Here's how the part is built. I have some questions about the finished solid (model axes, mm). Face numbers are marked on the shaded views. A direction names the side the tool comes from. Coordinates: 2 decimals unless noted, no trailing zeros. Write each loop counter-clockwise with the first axis right and the second up, starting at its lowest first coordinate (ties: lowest second). Pieces come first, ordered by that corner, then holes. Notation, with made-up numbers: M -17,20.5 L 38,20.5 A15 cw 38,44.5 Z; hole C -28.5,42 d2. An arc over 180 degrees is marked long. Use one line per item in the form item = value. Start each with the question number.
1. On a 3-axis mill with a long thin cutter (end or side, diameter ignored), from which of +Z, -Z, +X, -X, +Y, -Y can I reach the whole of each face in a straight line? I mean the marked faces 1, 2 and 3. Say none if no direction works.
2. Please list where these lines run through material, in increasing order: line 1 along Z through (x, y) = (10, 2.3); line 2 along X through (y, z) = (1.6, 13.5); line 3 along Z through (x, y) = (-9, 2.7). Write a range as [from, to].
3. I want a section at A-A, the plane z = -13.5. Count the separate pieces of the cut face and the enclosed holes in it, plus the area to 3 significant figures.
4. I want a section at B-B, the plane x = -9.75. List the corners of the cut face in (y, z) for me, plus the area to 3 significant figures.
5. I want a section at D-D, the plane x = 13.5. List the corners of the cut face in (y, z) for me.
6. I'm going to push flat-ended pins straight in: pin 1 Ø3 at (x, z) = (7.5, -5.5) entering from +Y; pin 2 Ø4.5 at (x, z) = (10, -13.5) entering from -Y. Where does each tip first touch, or does it pass through?
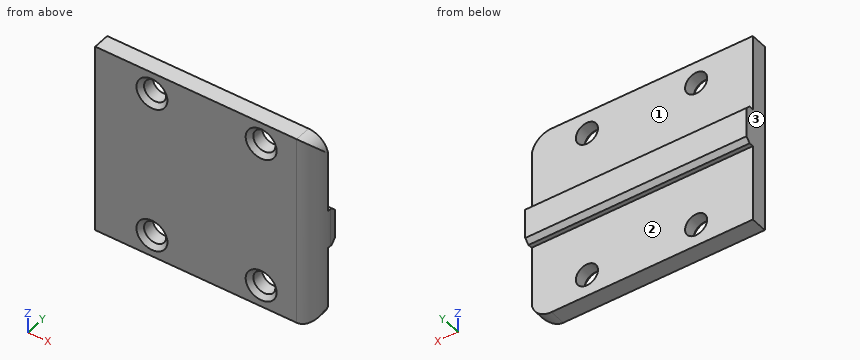
Autodesk Inventor part; units mm, degrees
ref_plane "YZ Plane" through (0, 0, 0) normal (1, 0, 0) x (0, 1, 0)
ref_plane "XZ Plane" through (0, 0, 0) normal (0, 1, 0) x (-1, 0, 0)
ref_plane "XY Plane" through (0, 0, 0) normal (0, 0, 1) x (1, 0, 0)
sketch "Sketch2" plane through (0, 0, 0) normal (0, 1, 0) x (-1, 0, 0)
  line L0 (20, 17.5) -> (-20, 17.5)
  line L1 (-20, 17.5) -> (-20, -17.5)
  line L2 (-20, -17.5) -> (20, -17.5)
  line L3 (20, -17.5) -> (20, 17.5)
  point P0 (0, 0)
  point P1 (20, 0)
  point P2 (0, -17.5)
  dimension "d0" = 40
  dimension "d1" = 35
extrude "Extrusion1" add sketch "Sketch2" along normal blind 3
sketch "Sketch3" plane through (0, 3, 0) normal (0, 1, 0) x (1, 0, 0)
  line L0 (-20, -17.5) -> (20, -17.5)
  line L1 (20, -17.5) -> (20, 17.5)
  line L2 (20, 17.5) -> (-20, 17.5)
  line L3 (-20, 17.5) -> (-20, -17.5)
  line L4 (-20, 0) -> (20, 0)
  line L5 (0, 0) -> (-9.75, 0)
  line L6 (-9.75, 0) -> (-9.75, 17.5)
  line L7 (0, 0) -> (9.75, 0)
  line L8 (9.75, 0) -> (9.75, 17.5)
  line L9 (0, 0) -> (0, 13.5)
  line L10 (0, 13.5) -> (-20, 13.5)
  line L11 (0, 13.5) -> (20, 13.5)
  circle A0 centre (10, 13.5) radius 2
  circle A1 centre (-9.75, 13.5) radius 2
  circle A2 centre (10, -13.5) radius 2
  circle A3 centre (-9.75, -13.5) radius 2
  dimension "d4" = 9.75
  dimension "d5" = 9.75
  dimension "d6" = 13.5
  dimension "d7" = 4
  dimension "d8" = 4
extrude "Extrusion2" cut sketch "Sketch3" against normal through all contours A1 L6 L10 | L10 L6 A1 | L6 L10 A1 | A0 L8 L11 | L11 L8 A0 | A0 L11 L8 | L6 A1 L10 | L11 A0 L8 | A2 | A3
sketch "Sketch4" plane through (0, 3, 0) normal (0, 1, 0) x (1, 0, 0)
  circle A0 centre (10, -13.5) radius 2
  circle A1 centre (-9.75, 13.5) radius 2
  circle A2 centre (10, 13.5) radius 2
  circle A3 centre (-9.75, -13.5) radius 2
  line L0 (-20, -17.5) -> (20, -17.5)
  line L1 (20, -17.5) -> (20, 17.5)
  line L2 (20, 17.5) -> (-20, 17.5)
  line L3 (-20, 17.5) -> (-20, -17.5)
  line L4 (20, -3.5) -> (-20, -3.5)
  line L5 (-20, -3.5) -> (-20, 3.5)
  line L6 (-20, 3.5) -> (20, 3.5)
  line L7 (20, 3.5) -> (20, -3.5)
  line L8 (20, -3.5) -> (-20, 3.5) construction
  line L9 (-20, -3.5) -> (20, 3.5) construction
  point P0 (0, 0)
  dimension "d11" = 7
extrude "Extrusion3" add sketch "Sketch4" along normal blind 1.6 contours L3 L6 L1 L4
fillet "Fillet1" radius 3.5875 3 edges at (20, 1.5, 17.5) (20, 1.5, -17.5) (20, 0, 0)
sketch "Sketch5" plane through (0, 0, 0) normal (0, -1, 0) x (1, 0, 0)
  circle A0 centre (-9.75, 13.5) radius 2
  circle A1 centre (10, -13.5) radius 2
  circle A2 centre (-9.75, -13.5) radius 2
  circle A3 centre (10, 13.5) radius 2
  line L0 (16.4125, 17.5) -> (16.4125, -17.5)
  line L1 (-20, 17.5) -> (16.4125, 17.5)
  line L2 (-20, -17.5) -> (-20, 17.5)
  line L3 (16.4125, -17.5) -> (-20, -17.5)
  circle A4 centre (-9.75, 13.5) radius 3
  circle A5 centre (10, 13.5) radius 3
  circle A6 centre (10, -13.5) radius 3
  circle A7 centre (-9.75, -13.5) radius 3
  point P0 (0, 0)
  dimension "d15" = 1
  dimension "d16" = 1
  dimension "d17" = 1
  dimension "d18" = 1
chamfer "Chamfer1" distance 0.8 angle 45 4 edges at (-11.75, 0, -13.5) (-11.75, 0, 13.5) (8, 0, 13.5) (8, 0, -13.5)
chamfer "Chamfer2" distance 0.8 angle 45 2 edges at (0, 4.6, 3.5) (0, 4.6, -3.5)
properties part number "RearCarriageSupport" material "ABS Plastic"
Answer list:
q1.face_1 = +Z, +X, -X, +Y
q1.face_2 = -Z, +X, -X, +Y
q1.face_3 = +Z, -Z, -X, +Y, -Y
q2.line_1 = [-17.5, -15.5], [-11.5, 11.5], [15.5, 17.5]
q2.line_2 = [-20, -11.75], [-7.75, 8], [12, 19.4]
q2.line_3 = [-17.5, -15.35], [-11.65, 11.65], [15.35, 17.5]
q3.separate_pieces = 3
q3.enclosed_holes = 0
q3.area = 92.0 mm²
q4.outline = M 0,-17.5 L 3,-17.5 L 3,-15.5 L 0.8,-15.5 L 0,-16.3 Z; M 0,-10.7 L 0.8,-11.5 L 3,-11.5 L 3,-3.5 L 3.8,-3.5 L 4.6,-2.7 L 4.6,2.7 L 3.8,3.5 L 3,3.5 L 3,11.5 L 0.8,11.5 L 0,10.7 Z; M 0,16.3 L 0.8,15.5 L 3,15.5 L 3,17.5 L 0,17.5 Z
q4.area = 90.3 mm²
q5.outline = M 0,-17.5 L 3,-17.5 L 3,-3.5 L 3.8,-3.5 L 4.6,-2.7 L 4.6,2.7 L 3.8,3.5 L 3,3.5 L 3,17.5 L 0,17.5 Z
q6.pin_1 = 3
q6.pin_2 = 0.55
